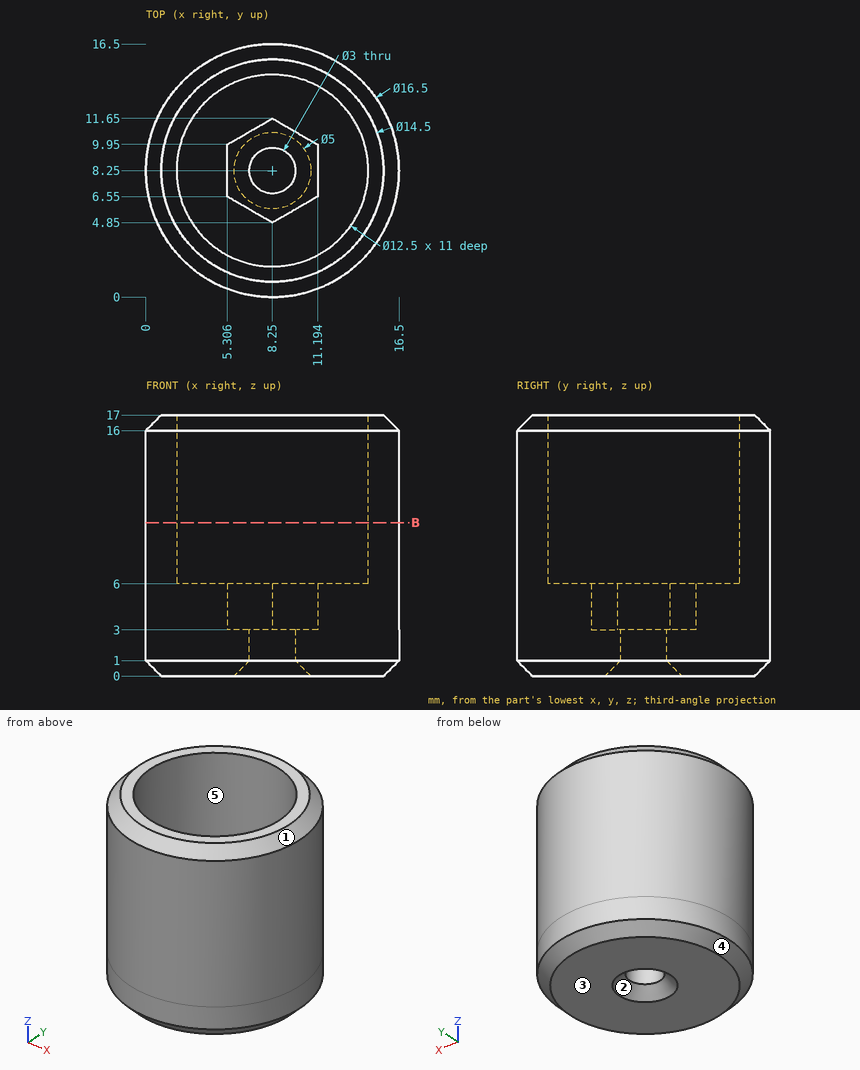
Could you check a few things on this drawing? It's one solid part, dimensions in mm from its lowest x, y, z. A direction names the side the tool comes from. Round coordinates to 2 decimals unless told otherwise and drop trailing zeros. Order: outer loops, then holes, each group sorted by start corner. A loop starts at its lowest first (then second) coordinate and runs counter-clockwise, first axis right, second up. Notation, with made-up numbers: M 87,65.25 L 115,65.25 A22 ccw 115,84.25 Z; hole C 8.5,41.5 d8. An arc over 180 degrees is marked long. Use a Markdown table: item, result.
1) If we mould it in two halves opening along X, with no side actions, what happens to the marked faces 1, 2 and 3? For each: +X half, -X half, draft (parallel to the pull), parting line (faces both ways), or undercut.
Geometry says:
| item | result |
|---|---|
| face 1 | parting line |
| face 2 | undercut |
| face 3 | draft |
2) Imagine slicing it at B-B (z = 10). List the corners of the cut face in (x, y) for me.
Geometry says:
| item | result |
|---|---|
| outline | C 8.25,8.25 d16.5; hole C 8.25,8.25 d12.5 |
3) On a 3-axis mill with a long thin cutter (end or side, diameter ignored), from which of +Z, -Z, +X, -X, +Y, -Y can I reach the whole of each face in a straight line? I mean the marked faces 4 and 5. Say none if no direction works.
Geometry says:
| item | result |
|---|---|
| face 4 | -Z |
| face 5 | +Z |
4) If I drill on line 1 along X through (y, z) = (8, 11.5) (1 decimal); line 2 along Y through (x, z) = (8.25, 1.85), over which ranges is the centre line in solid material (lowest first)?
Geometry says:
| item | result |
|---|---|
| line 1 | x = 0 to 2, 14.5 to 16.5 |
| line 2 | y = 0 to 6.75, 9.75 to 16.5 |
5) I'm going to push flat-ended pins straight in: P1, Ø6, axis at y = 8.5, z = 6.5, coming from the -X side; P2, Ø8, axis at y = 13.5, z = 7.5, coming from the +X side (1 decimal); P3, Ø3, axis at x = 2, z = 7.5, coming from the -Y side (1 decimal); P4, Ø5, axis at y = 4.5, z = 11.5, coming from the -X side (1 decimal). Where does each tip first touch, or does it pass through?
Geometry says:
| item | result |
|---|---|
| P1 | stops at x = 0 |
| P2 | stops at x = 16.4 |
| P3 | stops at y = 1.5 |
| P4 | stops at x = 0.1 |
